```python
from build123d import *

# Parameters (mm, degrees)
F1_DEPTH        = 25.4
F2_R            = 13.49375
F3_DEPTH        = 25.4
F4_R            = 30.99943
F4_R_2          = 13.49375
F5_DEPTH        = 17.78
F6_R            = 31.0007
F6_R_2          = 12.50061
F7_DEPTH        = 16.99768
F8_DEPTH        = 16.99768
F11_D           = 6.35
F11_DEPTH       = 38.1
F11_CBORE_D     = 12.7
F11_CBORE_DEPTH = 6.35
F11_TIP         = 1.9077324654
F13_D           = 6.35
F13_DEPTH       = 38.1
F13_CBORE_D     = 12.7
F13_CBORE_DEPTH = 6.35
F13_TIP         = 1.9077324654


# Not quite as in the source:
# - a feature names something its author has since deleted; it is built from what else it names


with BuildPart() as f1:
    # F0 (on Top) → F1 (new body)
    with BuildSketch(Plane.XY):
        with BuildLine():
            ThreePointArc((-50.8, -44.45), (-48.9401280605, -48.9401280605), (-44.45, -50.8))
            Line((-44.45, -50.8), (-31.75, -50.8))
            Line((-31.75, -50.8), (31.75, -50.8))
            Line((31.75, -50.8), (44.45, -50.8))
            ThreePointArc((44.45, -50.8), (48.9401280605, -48.9401280605), (50.8, -44.45))
            Line((50.8, -44.45), (50.8, 44.45))
            ThreePointArc((50.8, 44.45), (48.9401280605, 48.9401280605), (44.45, 50.8))
            Line((44.45, 50.8), (-44.45, 50.8))
            ThreePointArc((-44.45, 50.8), (-48.9401280605, 48.9401280605), (-50.8, 44.45))
            Line((-50.8, 44.45), (-50.8, -44.45))
        make_face()
    extrude(amount=F1_DEPTH)

    # F2 (on face) → F3 (cut)
    with BuildSketch(Plane.XY.offset(25.4)):
        Circle(F2_R)
    extrude(amount=-F3_DEPTH, mode=Mode.SUBTRACT)

    # F4 (on face) → F5 (cut)
    with BuildSketch(Plane.XY.offset(25.4)):
        Circle(F4_R)
        Circle(F4_R_2, mode=Mode.SUBTRACT)
    extrude(amount=-F5_DEPTH, mode=Mode.SUBTRACT)

    # F11
    with Locations(Plane(origin=(0, 0, 0), x_dir=(1, 0, 0), z_dir=(0, 0, -1))):
        with Locations((-21.59, -41.275), (21.59, -41.275), (-21.59, 41.275), (21.59, 41.275)):
            CounterBoreHole(F11_D / 2, F11_CBORE_D / 2, F11_CBORE_DEPTH, depth=F11_DEPTH)
            with Locations((0, 0, -(F11_DEPTH + F11_TIP / 2))):  # 118° drill point
                Cone(0, F11_D / 2, F11_TIP, mode=Mode.SUBTRACT)

    # F13
    with Locations(Plane.XY.offset(25.4)):
        with Locations((-41.275, 23.8990909091), (-41.275, -19.2809090909), (41.275, 23.8990909091), (41.275, -19.2809090909)):
            CounterBoreHole(F13_D / 2, F13_CBORE_D / 2, F13_CBORE_DEPTH, depth=F13_DEPTH)
            with Locations((0, 0, -(F13_DEPTH + F13_TIP / 2))):  # 118° drill point
                Cone(0, F13_D / 2, F13_TIP, mode=Mode.SUBTRACT)


with BuildPart() as f7:
    # F6 (on Top) → F7 (new body)
    with BuildSketch(Plane.XY):
        with Locations((-113.8032615222, 0)):
            Circle(F6_R)
        with Locations((-113.8032615222, 0)):
            Circle(F6_R_2, mode=Mode.SUBTRACT)
    extrude(amount=F7_DEPTH)


with BuildPart() as f8:
    # F6 (on Top) → F8 (new body)
    with BuildSketch(Plane.XY):
        with Locations((-113.8032615222, 0)):
            Circle(F6_R)
        with Locations((-113.8032615222, 0)):
            Circle(F6_R_2, mode=Mode.SUBTRACT)
    extrude(amount=F8_DEPTH)


solid = f1.part
```
Input: part model. Units: mm. Frame: model coordinates. A direction names the side the tool comes from. Coordinates: 2 decimals unless noted, no trailing zeros. Write each loop counter-clockwise with the first axis right and the second up, starting at its lowest first coordinate (ties: lowest second). Pieces come first, ordered by that corner, then holes.
1) Pin query (flat end, axial travel): pin 1 Ø8.5 at (x, y) = (21.59, 41.275) entering from -Z; pin 2 Ø6.5 at (x, y) = (39, -18.5) entering from +Z; pin 3 Ø18.5 at (x, y) = (-14.5, -8.5) entering from +Z. Return the tip coordinate at first contact, or that it passes through.
2) Section C-C on y = -8.5. Output: boundary loops of the cut face in (x, z).
3) Mould query, pull axis X, two halves, no side actions, for faces 4 (the flat face through (50.8, -1, 13)), 5 (the cylindrical face through (-48.99, -48.89, 12.52)), 6 (the flat face through (-23, 23, 25.4)), 7 (the cylindrical face through (39.9, -25.48, 22.27)). Classes: pulls with the +X half, pulls with the -X half, needs draft (parallel to the pull), parting line crosses it, or undercut.
4) Section B-B on x = -21.59. Output: boundary loops of the cut face in (y, z) (3 decimals), and give its area (3 significant figures).
5) Section A-A on x = 0. Output: boundary loops of the cut face in (y, z), and give its area (3 significant figures).
6) Section D-D on z = 16.5. State how many separate pieces and enclosed holes the cut face has, and give its area (3 significant figures).
7) Set-up query: faces 1 (the cylindrical face through (-38.93, 26.04, 9.39)), 2 (the flat face through (23, 38, 6.35)), 3 (the flat face through (13, -6, 7.62)). Return all of +Z, -Z, +X, -X, +Y, -Y with unobstructed straight access to the full face (end or side cutting, diameter ignored); none if empty.
8) Material intervals for line 1 along Y through (x, z) = (-21.59, 5) (3 decimals); line 2 along Y through (x, z) = (43.5, 23.75); line 3 along X through (y, z) = (21, 14.5), sorted ascending.
Check result:
1. pin 1: stops at z = 6.35
1. pin 2: stops at z = 19.05
1. pin 3: stops at z = 7.62
2. outline: (-50.8, 0) - (-10.48, 0) - (-10.48, 7.62) - (-29.81, 7.62) - (-29.81, 25.4) - (-50.8, 25.4) - close; (10.48, 0) - (50.8, 0) - (50.8, 25.4) - (29.81, 25.4) - (29.81, 7.62) - (10.48, 7.62) - close
3. face 4: pulls with the +X half
3. face 5: pulls with the -X half
3. face 6: needs draft
3. face 7: undercut
4. outline: (-50.8, 0) - (-47.625, 0) - (-47.625, 6.35) - (-44.45, 6.35) - (-44.45, 25.4) - (-50.8, 25.4) - close; (-38.1, 6.35) - (-34.925, 6.35) - (-34.925, 0) - (34.925, 0) - (34.925, 6.35) - (38.1, 6.35) - (38.1, 25.4) - (22.245, 25.4) - (22.245, 7.62) - (-22.245, 7.62) - (-22.245, 25.4) - (-38.1, 25.4) - close; (44.45, 6.35) - (47.625, 6.35) - (47.625, 0) - (50.8, 0) - (50.8, 25.4) - (44.45, 25.4) - close
4. area: 1,390 mm2
5. outline: (-50.8, 0) - (-13.49, 0) - (-13.49, 7.62) - (-31, 7.62) - (-31, 25.4) - (-50.8, 25.4) - close; (13.49, 0) - (50.8, 0) - (50.8, 25.4) - (31, 25.4) - (31, 7.62) - (13.49, 7.62) - close
5. area: 1,270 mm2
6. separate pieces: 1
6. enclosed holes: 9
6. area: 7,020 mm2
7. face 1: +Z, -Z
7. face 2: -Z
7. face 3: +Z
8. line 1: y = -50.8 to -47.625, -34.925 to 34.925, 47.625 to 50.8
8. line 2: y = -50.8 to -25.23, -13.33 to 17.95, 29.85 to 50.8
8. line 3: x = -50.8 to -42.57, -39.98 to -22.8, 22.8 to 39.98, 42.57 to 50.8
